from build123d import *
from build123d.topology import SkipClean

# Parameters (mm, degrees)
SKETCH1_W           = 101.6
SKETCH1_H           = 76.2
BOSS_EXTRUDE1_DEPTH = 30.48
SKETCH2_R           = 25.4
BOSS_EXTRUDE2_DEPTH = 12.7
SKETCH3_W           = 76.2
SKETCH3_H           = 76.2
CUT_EXTRUDE1_DEPTH  = 22.86
SKETCH5_R           = 25.4
CUT_EXTRUDE3_DEPTH  = 256.032
SKETCH6_R           = 1.45
CUT_EXTRUDE4_DEPTH  = 256.032


with BuildPart() as part:
    # Sketch1 → Boss-Extrude1 (new body)
    with BuildSketch(Plane(origin=(0, 0, 0), x_dir=(1, 0, 0), z_dir=(0, 1, 0))):
        Rectangle(SKETCH1_W, SKETCH1_H)
    extrude(amount=-BOSS_EXTRUDE1_DEPTH)

    # Sketch2 → Boss-Extrude2 (add)
    with BuildSketch(Plane.ZY.offset(50.8)):
        with BuildLine():
            Line((-38.1, -30.48), (38.1, -30.48))
            Line((38.1, -30.48), (38.1, 20.32))
            ThreePointArc((38.1, 20.32), (30.660512242, 38.280512242), (12.7, 45.72))
            Line((12.7, 45.72), (-12.7, 45.72))
            ThreePointArc((-12.7, 45.72), (-30.660512242, 38.280512242), (-38.1, 20.32))
            Line((-38.1, 20.32), (-38.1, -30.48))
        make_face()
        with Locations((0, 7.62)):
            Circle(SKETCH2_R, mode=Mode.SUBTRACT)
    boss_extrude2 = extrude(amount=-BOSS_EXTRUDE2_DEPTH)

    # Mirror1: Boss-Extrude2 across plane
    add(boss_extrude2.mirror(Plane(origin=(0, 0, 0), x_dir=(0, 0, 1), z_dir=(1, 0, 0))))

    # Sketch3 → Cut-Extrude1 (cut)
    with BuildSketch(Plane(origin=(0, 0, 0), x_dir=(1, 0, 0), z_dir=(0, 1, 0))):
        Rectangle(SKETCH3_W, SKETCH3_H)
    extrude(amount=-CUT_EXTRUDE1_DEPTH, mode=Mode.SUBTRACT)

    # Sketch5 → Cut-Extrude3 (cut)
    with SkipClean():  # the faces are left unmerged after this step: merging them gives an invalid solid
        with BuildSketch(Plane.ZY.offset(50.8)):
            with Locations((0, 7.62)):
                Circle(SKETCH5_R)
        extrude(amount=-CUT_EXTRUDE3_DEPTH, mode=Mode.SUBTRACT)

    # Sketch6 → Cut-Extrude4 (cut)
    with SkipClean():  # the faces are left unmerged after this step: merging them gives an invalid solid
        with BuildSketch(Plane(origin=(0, -22.86, 0), x_dir=(1, 0, 0), z_dir=(0, 1, 0))):
            with Locations(Location((-27.94, 27.94, 0), (0, 0, 270))):
                Circle(SKETCH6_R)
            with Locations(Location((27.94, 27.94, 0), (0, 0, 90))):
                Circle(SKETCH6_R)
            with Locations(Location((27.94, -27.94, 0), (0, 0, 270))):
                Circle(SKETCH6_R)
            with Locations(Location((-27.94, -27.94, 0), (0, 0, 90))):
                Circle(SKETCH6_R)
        extrude(amount=-CUT_EXTRUDE4_DEPTH, mode=Mode.SUBTRACT)


solid = part.part
Build history of the part. All positions in model axes, mm. A direction names the side the tool comes from. Give positions to 0.01 mm unless a question says otherwise; leave off trailing zeros. Write each loop counter-clockwise with the first axis right and the second up, starting at its lowest first coordinate (ties: lowest second). Pieces come first, ordered by that corner, then holes. Notation, with made-up numbers: (13, -19) - (64, -19) arc R14 ccw to (64, 4) - close; hole circle Ø2 at (14, -4). An arc over 180 degrees is marked (long way). Use one line per item in the form item = value. Start each with the question number.
1. Drop flat-ended pins along their axis: pin 1 Ø4.5 at (x, z) = (27.94, 27.94) entering from +Y; pin 2 Ø4 at (x, z) = (-27.94, -27.94) entering from -Y. Give the stop position or say it passes through.
2. 3-axis set-ups, long thin cutter, end or side, ignore diameter. For faces 5 (the face through (50.8, -17, -8)), 6 (the face through (-1, -22.86, -1)): which of +Z, -Z, +X, -X, +Y, -Y reach the whole face in a straight line?
3. Band-saw the part on A-A on z = 0. Write the cut outline in (x, y), plus the area to 3 significant figures.
4. Two-plate mould, pull along Z, no slides. Class faces 1 (the face through (44.54, 38.48, -30.46)), 2 (the face through (45, 45.72, 0)), 3 (the face through (-29.226, -26.617, -27.271)), 4 (the face through (28.495, -26.617, -29.279)): released by +Z, released by -Z, zero draft, split by the parting line, or undercut.
5. Band-saw the part on C-C on y = 2.5. Write the cut outline in (x, z).
6. Band-saw the part on B-B on x = -27.94. Write the cut outline in (y, z).
7. Probe line 1 (X direction, y = -28, z = 27.94); line 2 (X direction, y = 4.5, z = 32.5); line 3 (Y direction, x = -44.5, z = 0). List the from-to ranges inside material, lowest first. Write a range as [from, to].
8. Band-saw the part on D-D on y = 34.5. Write the cut outline in (x, z).
Conclusion:
q1.pin_1 = -22.86
q1.pin_2 = -30.48
q2.face_5 = +Z, -Z, +X, +Y, -Y
q2.face_6 = +Z, -Z, +Y
q3.outline = (-50.8, -30.48) - (50.8, -30.48) - (50.8, -17.78) - (38.1, -17.78) - (38.1, -22.86) - (-38.1, -22.86) - (-38.1, -17.78) - (-50.8, -17.78) - close; (-50.8, 33.02) - (-38.1, 33.02) - (-38.1, 45.72) - (-50.8, 45.72) - close; (38.1, 33.02) - (50.8, 33.02) - (50.8, 45.72) - (38.1, 45.72) - close
q3.area = 1,230 mm²
q4.face_1 = released by -Z
q4.face_2 = zero draft
q4.face_3 = undercut
q4.face_4 = undercut
q5.outline = (-50.8, -38.1) - (-38.1, -38.1) - (-38.1, -24.88) - (-50.8, -24.88) - close; (-50.8, 24.88) - (-38.1, 24.88) - (-38.1, 38.1) - (-50.8, 38.1) - close; (38.1, -38.1) - (50.8, -38.1) - (50.8, -24.88) - (38.1, -24.88) - close; (38.1, 24.88) - (50.8, 24.88) - (50.8, 38.1) - (38.1, 38.1) - close
q6.outline = (-30.48, -38.1) - (-22.86, -38.1) - (-22.86, -29.39) - (-30.48, -29.39) - close; (-30.48, -26.49) - (-22.86, -26.49) - (-22.86, 26.49) - (-30.48, 26.49) - close; (-30.48, 29.39) - (-22.86, 29.39) - (-22.86, 38.1) - (-30.48, 38.1) - close
q7.line_1 = [-50.8, -29.39], [-26.49, 26.49], [29.39, 50.8]
q7.line_2 = [-50.8, -38.1], [38.1, 50.8]
q7.line_3 = [-30.48, -17.78], [33.02, 45.72]
q8.outline = (-50.8, -33.77) - (-38.1, -33.77) - (-38.1, 33.77) - (-50.8, 33.77) - close; (38.1, -33.77) - (50.8, -33.77) - (50.8, 33.77) - (38.1, 33.77) - close
